```python
from build123d import *

# Parameters (mm, degrees)
SKETCH_1_W          = 27.8
SKETCH_1_H          = 27.8
SKETCH_1_R          = 5.5
EXTRUDE_1_DEPTH     = 5
SKETCH_1_15_R       = 1.5
CUT_EXTRUDE_1_DEPTH = 32.480946619
SKETCH_1_16_R       = 2.25
CUT_EXTRUDE_2_DEPTH = 3
SKETCH_2_R          = 0.75
CUT_EXTRUDE_3_DEPTH = 4
CUT_EXTRUDE_START   = -23.8
SKETCH_2_3_R        = 0.75
CUT_EXTRUDE_4_DEPTH = 4
SKETCH_3_R          = 0.75
CUT_EXTRUDE_5_DEPTH = 4
SKETCH_3_3_R        = 0.75
CUT_EXTRUDE_6_DEPTH = 4


with BuildPart() as part:
    # 草图1 → 凸台-拉伸1 (new body)
    with BuildSketch(Plane(origin=(0, 0, 0), x_dir=(1, 0, 0), z_dir=(0, 1, 0))):
        with Locations((13.9, 0)):
            Rectangle(SKETCH_1_W, SKETCH_1_H)
        with Locations(Location((13.9, 0, 0), (0, 0, 270))):
            Circle(SKETCH_1_R, mode=Mode.SUBTRACT)
    extrude(amount=EXTRUDE_1_DEPTH)

    # 草图1<15> → 切除-拉伸1 (cut, through all)
    with BuildSketch(Plane(origin=(0, 0, 0), x_dir=(1, 0, 0), z_dir=(0, 1, 0))):
        with Locations(Location((5.9, 0, 0), (0, 0, 270))):
            Circle(SKETCH_1_15_R)
        with Locations(Location((21.9, 0, 0), (0, 0, 270))):
            Circle(SKETCH_1_15_R)
    extrude(amount=CUT_EXTRUDE_1_DEPTH, mode=Mode.SUBTRACT)

    # 草图1<16> → 切除-拉伸2 (cut)
    with BuildSketch(Plane(origin=(0, 0, 0), x_dir=(1, 0, 0), z_dir=(0, 1, 0))):
        with Locations(Location((5.9, 0, 0), (0, 0, 90))):
            Circle(SKETCH_1_16_R)
        with Locations(Location((21.9, 0, 0), (0, 0, 90))):
            Circle(SKETCH_1_16_R)
    extrude(amount=CUT_EXTRUDE_2_DEPTH, mode=Mode.SUBTRACT)

    # 草图2 → 切除-拉伸3 (cut)
    with BuildSketch(Plane(origin=(0, 0, -13.9), x_dir=(-1, 0, 0), z_dir=(0, 0, -1))):
        with Locations((-22.8, 2.5)):
            Circle(SKETCH_2_R)
        with Locations((-5, 2.5)):
            Circle(SKETCH_2_R)
    extrude(amount=-CUT_EXTRUDE_3_DEPTH, mode=Mode.SUBTRACT)

    # 草图2<3> → 切除-拉伸4 (cut)
    with BuildSketch(Plane(origin=(0, 0, -13.9), x_dir=(-1, 0, 0), z_dir=(0, 0, -1)).offset(CUT_EXTRUDE_START)):
        with Locations((-22.8, 2.5)):
            Circle(SKETCH_2_3_R)
        with Locations((-5, 2.5)):
            Circle(SKETCH_2_3_R)
    extrude(amount=-CUT_EXTRUDE_4_DEPTH, mode=Mode.SUBTRACT)

    # 草图3 → 切除-拉伸5 (cut)
    with BuildSketch(Plane.ZY):
        with Locations((-8.9, 2.5)):
            Circle(SKETCH_3_R)
        with Locations((8.9, 2.5)):
            Circle(SKETCH_3_R)
    extrude(amount=-CUT_EXTRUDE_5_DEPTH, mode=Mode.SUBTRACT)

    # 草图3<3> → 切除-拉伸6 (cut)
    with BuildSketch(Plane.ZY.offset(CUT_EXTRUDE_START)):
        with Locations((-8.9, 2.5)):
            Circle(SKETCH_3_3_R)
        with Locations((8.9, 2.5)):
            Circle(SKETCH_3_3_R)
    extrude(amount=-CUT_EXTRUDE_6_DEPTH, mode=Mode.SUBTRACT)


solid = part.part
```
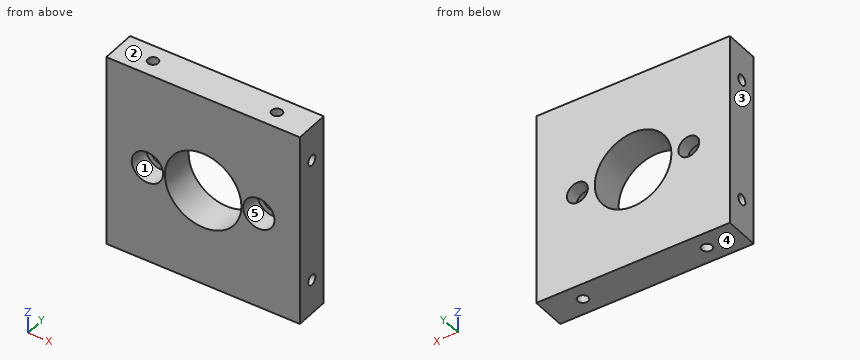
Verification items for the finished model (mm, model axes). Face numbers are marked on the shaded views. A direction names the side the tool comes from. Round coordinates to 2 decimals unless told otherwise and drop trailing zeros. Order: outer loops, then holes, each group sorted by start corner. A loop starts at its lowest first (then second) coordinate and runs counter-clockwise, first axis right, second up. Notation, with made-up numbers: (39.25, 55.25) -> (89.25, 55.25) arc R8 ccw to (89.25, 62.25) -> close; hole circle Ø11 at (64, 9). An arc over 180 degrees is marked (long way). Put each result on its own line as item: value. Start each with the question number.
(1) Section check D-D (x = 13.9). Enter the section's corners in (y, z).
(2) Depth check by flat-ended pin: pin 1 Ø1.4 at (y, z) = (2.5, -8.9) entering from -X; pin 2 Ø9 at (x, z) = (13.9, 0) entering from -Y; pin 3 Ø2 at (x, z) = (6, 1) entering from -Y; pin 4 Ø1.4 at (x, y) = (22.8, 2.5) entering from +Z. Enter the tip coordinate at first touch or a pass-through.
(3) Tool access check on the marked faces 1 and 2. Record the directions out of +Z, -Z, +X, -X, +Y, -Y that give a thin tool (end or side, any length) a straight path to the whole face; none if there is none.
(4) Material ranges on line 1 along X through (y, z) = (1.4, 0); line 2 along X through (y, z) = (3.5, 0); line 3 along Z through (x, y) = (21.9, 3.7), recorded low to high.
(5) Section check A-A (x = 9.5). Enter the section's corners in (y, z).
(6) Section check B-B (y = 1). Enter the section's corners in (x, z).
(7) Draft check along X on the marked faces 3, 4 and 5. Enter one of: +X half, -X half, draft (parallel to the pull), parting line (faces both ways), or undercut.
(8) Section check C-C (z = -12). Enter the section's corners in (x, y).
Completed:
1. outline: (0, -13.9) -> (5, -13.9) -> (5, -5.5) -> (0, -5.5) -> close; (0, 5.5) -> (5, 5.5) -> (5, 13.9) -> (0, 13.9) -> close
2. pin 1: stops at x = 4
2. pin 2: passes through
2. pin 3: stops at y = 3
2. pin 4: stops at z = 9.9
3. face 1: -Y
3. face 2: +Z, +X, -X, +Y, -Y
4. line 1: x = 0 to 3.65, 8.15 to 8.4, 19.4 to 19.65, 24.15 to 27.8
4. line 2: x = 0 to 4.4, 7.4 to 8.4, 19.4 to 20.4, 23.4 to 27.8
4. line 3: z = -13.9 to -1.5, 1.5 to 13.9
5. outline: (0, -13.9) -> (5, -13.9) -> (5, -3.3) -> (0, -3.3) -> close; (0, 3.3) -> (5, 3.3) -> (5, 13.9) -> (0, 13.9) -> close
6. outline: (0, -13.9) -> (27.8, -13.9) -> (27.8, 13.9) -> (0, 13.9) -> close; hole circle Ø4.5 at (5.9, 0); hole circle Ø11 at (13.9, 0); hole circle Ø4.5 at (21.9, 0)
7. face 3: -X half
7. face 4: draft
7. face 5: undercut
8. outline: (0, 0) -> (27.8, 0) -> (27.8, 5) -> (0, 5) -> close; hole circle Ø1.5 at (5, 2.5); hole circle Ø1.5 at (22.8, 2.5)
